Could you check a few things on this drawing? It's one solid part, dimensions in mm from its lowest x, y, z. A direction names the side the tool comes from. Give positions to 0.01 mm unless a question says otherwise; leave off trailing zeros. Loops run counter-clockwise (first coordinate to the right, second up) from the corner with the lowest first, then second, coordinate; pieces in that order, holes last. Notation, with made-up numbers: M -20.5,26 L -16.5,26 A13 ccw -16.5,34 Z; hole C 70.25,-5.75 d8. An arc over 180 degrees is marked long. Answer in a Markdown table with one row per item. Add a question column.
1. If we section it at D-D on z = 1: List the corners of the cut face in (x, y) for me.
2. I'm going to push flat-ended pins straight in: pin 1 Ø1 at (x, y) = (4.5, 22) entering from +Z; pin 2 Ø4.5 at (y, z) = (27.5, 7.5) entering from -X (1 decimal); pin 3 Ø1.6 at (x, z) = (3.5, 7) entering from -Y. Where does each tip first touch, or does it pass through?
3. I need wall thicknesses on line 1 along Z through (x, y) = (3.2, 29); line 2 along Y through (x, z) = (3.8, 11.25); line 3 along Z through (x, y) = (3.85, 14.5). Which ranges of each line are inside material? Lowest first, please. Write a range as from..to.
4. If we section it at A-A on z = 10: List the corners of the cut face in (x, y) for me, then the cut area to 3 significant figures.
5. If we section it at C-C on x = 4.3: List the corners of the cut face in (y, z) for me.
6. Which directions (+Z, -Z, +X, -X, +Y, -Y) give clear straight access to the entire face, cutting with the end or side of a thin tool? Please do the marked faces 1, 2, 3, 4 and 5.
7. If we section it at B-B on y = 24: List the corners of the cut face in (x, z) for me, then the cut area to 3 significant figures.
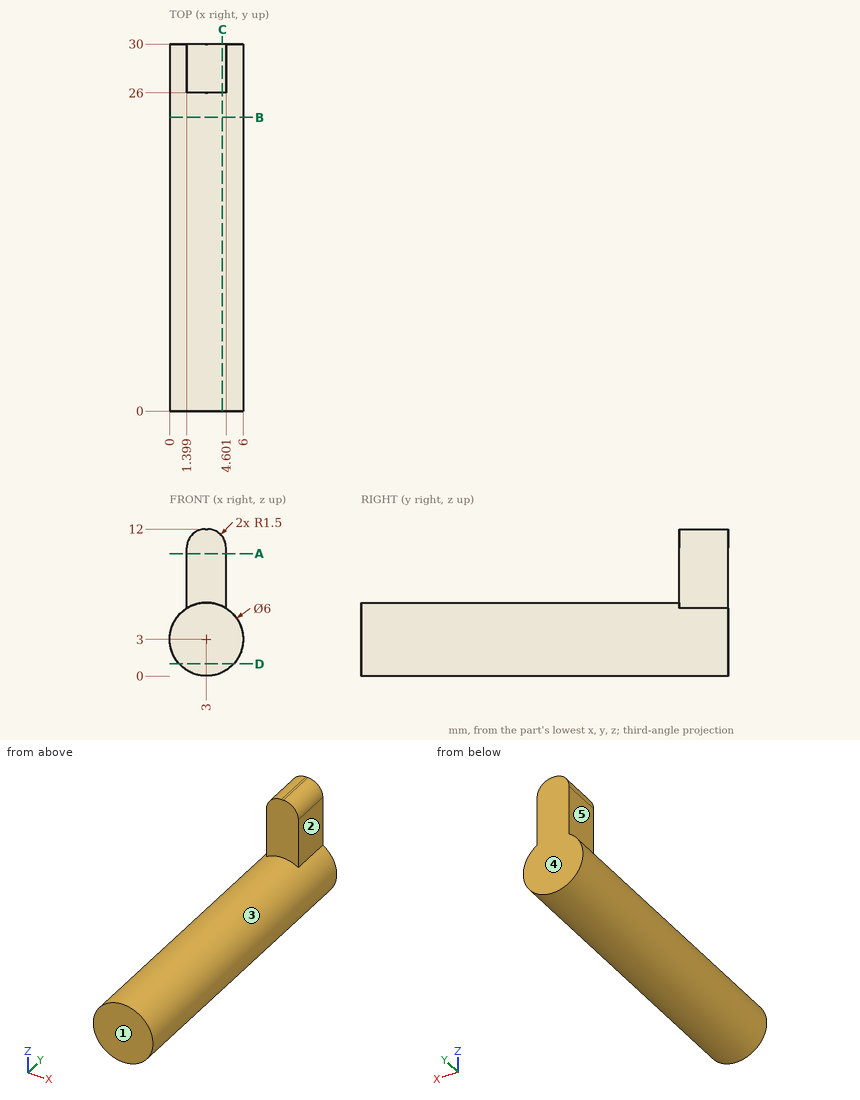
Results:
| question | item | result |
|---|---|---|
| 1 | outline | M 0.76,0 L 5.24,0 L 5.24,30 L 0.76,30 Z |
| 2 | pin 1 | z = 5.83 |
| 2 | pin 2 | x = 1 |
| 2 | pin 3 | y = 26 |
| 3 | line 1 | 0.01..12 |
| 3 | line 2 | 26..30 |
| 3 | line 3 | 0.12..5.88 |
| 4 | outline | M 1.4,26 L 4.6,26 L 4.6,30 L 1.4,30 Z |
| 4 | area | 12.8 mm2 |
| 5 | outline | M 0,0.3 L 30,0.3 L 30,11.4 L 26,11.4 L 26,5.7 L 0,5.7 Z |
| 6 | face 1 | +Z, -Z, +X, -X, -Y |
| 6 | face 2 | +Z, +X, +Y, -Y |
| 6 | face 3 | -Y |
| 6 | face 4 | +Z, -Z, +X, -X, +Y |
| 6 | face 5 | +Z, -X, +Y, -Y |
| 7 | outline | C 3,3 d6 |
| 7 | area | 28.3 mm2 |
